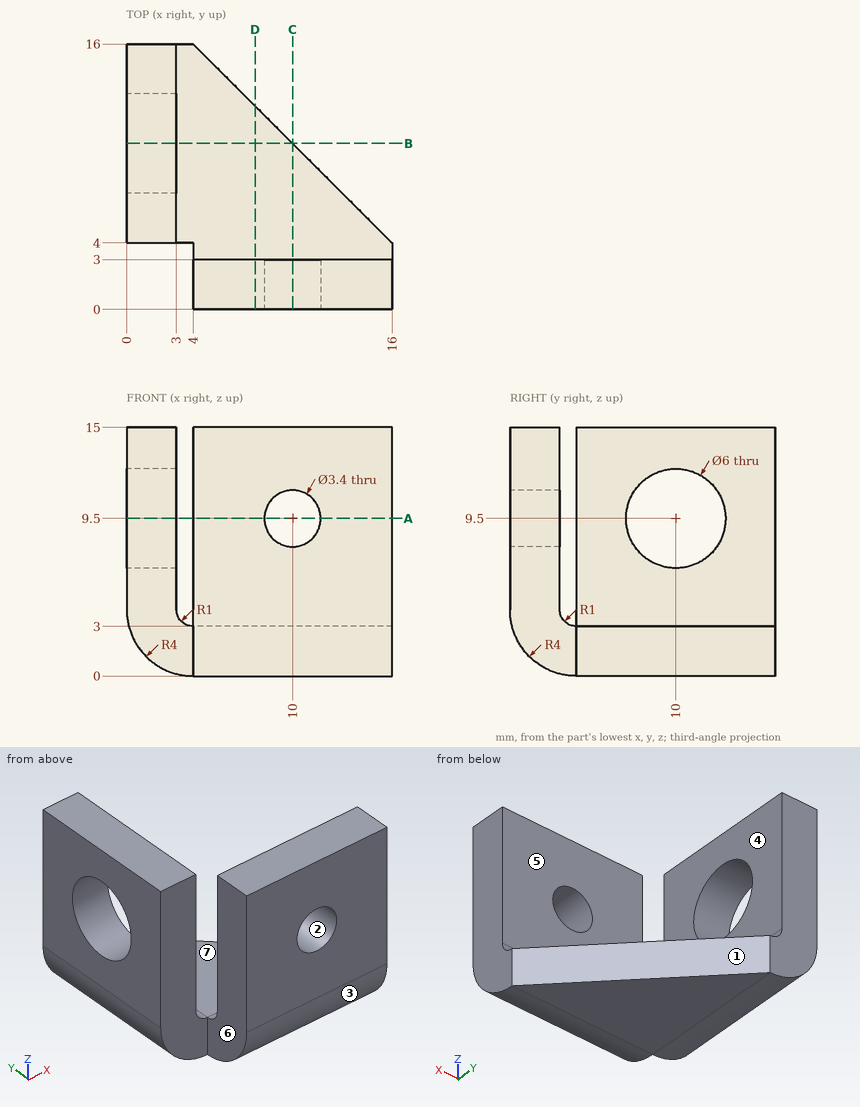
Geometry: see drawing. Coordinates: mm, zero at the bounding-box minimum. A direction names the side the tool comes from. Coordinates: 2 decimals unless noted, no trailing zeros. Loops run counter-clockwise (first coordinate to the right, second up) from the corner with the lowest first, then second, coordinate; pieces in that order, holes last. Notation, with made-up numbers: (-18.5, 35.5) -> (34.5, 35.5) arc R17 cw to (34.5, 62.5) -> close; hole circle Ø4 at (6, 2.5). An arc over 180 degrees is marked (long way). Use a Markdown table: item, result.
1) Cut plane D-D (x = 7.75). Return the cut outline in (y, z), then the cut area to 3 significant figures.
Results found:
| item | result |
|---|---|
| outline | (0, 4) arc R4 ccw to (4, 0) -> (12.25, 0) -> (12.25, 3) -> (4, 3) arc R1 cw to (3, 4) -> (3, 15) -> (0, 15) -> close |
| area | 69.5 mm2 |
2) Cut plane A-A (z = 9.5). Return the cut outline in (x, y).
Results found:
| item | result |
|---|---|
| outline | (0, 4) -> (3, 4) -> (3, 7) -> (0, 7) -> close; (0, 13) -> (3, 13) -> (3, 16) -> (0, 16) -> close; (4, 0) -> (8.3, 0) -> (8.3, 3) -> (4, 3) -> close; (11.7, 0) -> (16, 0) -> (16, 3) -> (11.7, 3) -> close |
3) Cut plane B-B (y = 10). Return the cut outline in (x, z), then the cut area to 3 significant figures.
Results found:
| item | result |
|---|---|
| outline | (0, 4) arc R4 ccw to (4, 0) -> (10, 0) -> (10, 3) -> (4, 3) arc R1 cw to (3, 4) -> (3, 6.5) -> (0, 6.5) -> close; (0, 12.5) -> (3, 12.5) -> (3, 15) -> (0, 15) -> close |
| area | 44.8 mm2 |
4) Access query for the marked faces 4, 5, 6 and 7. Directions: +Z, -Z, +X, -X, +Y, -Y. A direction counts if a zero-diameter tool reaches every point of the face in a straight line with its end or side. Return the directions, or none.
Results found:
| item | result |
|---|---|
| face 4 | +Z, +X, +Y, -Y |
| face 5 | +Z, +X, -X, +Y |
| face 6 | +Z, -Z, -X, -Y |
| face 7 | +Z, +X, +Y |
5) Pull-direction query (X, two-part tool) for the marked faces 1, 2 and 3; classes: released by +X, released by -X, zero draft, split by the parting line, or undercut.
Results found:
| item | result |
|---|---|
| face 1 | released by +X |
| face 2 | undercut |
| face 3 | zero draft |
6) Material intervals for line 1 along Y through (x, z) = (1.3, 9.5); line 2 along X through (y, z) = (1.15, 9.5); line 3 along X through (y, z) = (9.75, 14), sorted ascending. Write a range as from..to.
Results found:
| item | result |
|---|---|
| line 1 | y = 4..7, 13..16 |
| line 2 | x = 4..8.3, 11.7..16 |
| line 3 | x = 0..3 |
7) Contact query for flat-ended pins moving along their axis: pin 1 (8 mm diameter, centred on x = 5.5, y = 10.5, fed in from -Z); pin 2 (1.5 mm diameter, centred on y = 5, z = 12.5, fed in from +X); pin 3 (1.2 mm diameter, centred on y = 1, z = 9, fed in from -X); pin 4 (9 mm diameter, centred on y = 9.5, z = 8, fed in from +X). Output: stop coordinate, or through.
Results found:
| item | result |
|---|---|
| pin 1 | stops at z = 0 |
| pin 2 | stops at x = 3 |
| pin 3 | stops at x = 4 |
| pin 4 | stops at x = 3.13 |
8) Cut plane C-C (x = 10). Return the cut outline in (y, z).
Results found:
| item | result |
|---|---|
| outline | (0, 4) arc R4 ccw to (4, 0) -> (10, 0) -> (10, 3) -> (4, 3) arc R1 cw to (3, 4) -> (3, 7.8) -> (0, 7.8) -> close; (0, 11.2) -> (3, 11.2) -> (3, 15) -> (0, 15) -> close |
